Could you check a few things on this model? Use its own coordinates, in mm. A direction names the side the tool comes from. Coordinates: 2 decimals unless noted, no trailing zeros. Loops run counter-clockwise (first coordinate to the right, second up) from the corner with the lowest first, then second, coordinate; pieces in that order, holes last. Notation, with made-up numbers: M -28.5,-32 L -24.5,-32 A29 ccw -24.5,-7 Z; hole C -33.5,-5 d3. An arc over 180 degrees is marked long. Return JSON: item names as keys, results as strings. Group by question number.
from build123d import *

# Parameters (mm, degrees)
SKETCH1_R           = 100
BOSS_EXTRUDE1_DEPTH = 20
SKETCH2_R           = 12.5
SKETCH2_R_2         = 11.5
BOSS_EXTRUDE2_DEPTH = 60
CUT_EXTRUDE1_REACH  = 102
SKETCH3_R           = 1.5


with BuildPart() as part:
    # Sketch1 → Boss-Extrude1 (new body)
    with BuildSketch(Plane(origin=(0, 0, 0), x_dir=(1, 0, 0), z_dir=(0, 1, 0))):
        Circle(SKETCH1_R)
    extrude(amount=BOSS_EXTRUDE1_DEPTH)

    # Sketch2 → Boss-Extrude2 (add)
    with BuildSketch(Plane(origin=(0, 20, 0), x_dir=(1, 0, 0), z_dir=(0, 1, 0))):
        Circle(SKETCH2_R)
        Circle(SKETCH2_R_2, mode=Mode.SUBTRACT)
    extrude(amount=BOSS_EXTRUDE2_DEPTH)

    # Sketch3 → Cut-Extrude1 (cut, up to next)
    with BuildSketch(Plane.XY, mode=Mode.PRIVATE) as cut_extrude1_sk1:
        with Locations((0, 73.383174369)):
            Circle(SKETCH3_R)
    cut_extrude1_tool1 = extrude(cut_extrude1_sk1.sketch, amount=CUT_EXTRUDE1_REACH, mode=Mode.PRIVATE) & part.part
    add(cut_extrude1_tool1.solids().sort_by_distance((0, 73.383174, 0))[0], mode=Mode.SUBTRACT)


solid = part.part
(1) Imagine slicing it at D-D, the plane z = 49. Write out the boundary of the cut face in (x, y).
(2) For faces 4 (the face through (0, 20, 0)), 5 (the face through (95.38, 9.86, -30.04)), which set-ups out of +Z, -Z, +X, -X, +Y, -Y let a thin tool reach every point of the face, with its end or its side?
(3) Imagine slicing it at A-A, the plane z = 0. Write out the boundary of the cut face in (x, y).
(4) Imagine slicing it at C-C, the plane x = 46.5. Write out the boundary of the cut face in (y, z), then the cut area to 3 significant figures.
(5) Imagine slicing it at B-B, the plane y = 35. Write out the boundary of the cut face in (x, z).
(6) If I drill on L1, parallel to Z at x = 0, y = 50; L2, parallel to Y at x = 0, z = 12, over which ranges is the centre line in solid material (lowest first)? Write a range as [from, to].
(7) We'd pull the mould along X, two halves only. Please class faces 1 (the face through (-1, 0, -1)), 2 (the face through (11.923, 49.58, -3.755)), 3 (the face through (-1.5, 49.6, -11.4)): +X half, -X half, draft (parallel to the pull), parting line (faces both ways), or undercut.
(8) Will these pins go through, and if not, where does the flat tip stop? P1, Ø3, axis at x = 53, z = 31, coming from the +Y side; P2, Ø12, axis at x = 33.5, y = 23, coming from the +Z side; P3, Ø1, axis at y = 61.5, z = -6, coming from the -X side (3 decimals).
Checks:
{
 "1": {"outline": "M -87.17,0 L 87.17,0 L 87.17,20 L -87.17,20 Z"},
 "2": {"face 4": "+Y", "face 5": "+Y, -Y"},
 "3": {"outline": "M -100,0 L 100,0 L 100,20 L 12.5,20 L 12.5,80 L 11.5,80 L 11.5,20 L -11.5,20 L -11.5,80 L -12.5,80 L -12.5,20 L -100,20 Z"},
 "4": {"outline": "M 0,-88.53 L 20,-88.53 L 20,88.53 L 0,88.53 Z", "area": "3,540 mm²"},
 "5": {"outline": "C 0,0 d25; hole C 0,0 d23"},
 "6": {"L1": "[-12.5, -11.5], [11.5, 12.5]", "L2": "[0, 71.88], [74.88, 80]"},
 "7": {"face 1": "draft", "face 2": "parting line", "face 3": "undercut"},
 "8": {"P1": "y = 20", "P2": "z = 95.91", "P3": "x = -11.225"}
}
